```python
from build123d import *

# Parameters (mm, degrees)
REVOLVE1_ANGLE = 180


with BuildPart() as part:
    # Sketch1 → Revolve1 (revolve)
    with BuildSketch(Plane(origin=(0, 0, 0), x_dir=(1, 0, 0), z_dir=(0, 1, 0))):
        with BuildLine():
            Line((0, -6.35), (0, 6.35))
            Line((0, 6.35), (26.797, 6.35))
            ThreePointArc((26.797, 6.35), (27.695025612, 5.978025612), (28.067, 5.08))
            Line((28.067, 5.08), (28.067, 4.787411514))
            ThreePointArc((28.067, 4.787411514), (27.803594283, 4.013029212), (27.122641026, 3.5598701))
            ThreePointArc((27.122641026, 3.5598701), (24.384, 0), (27.122641026, -3.5598701))
            ThreePointArc((27.122641026, -3.5598701), (27.803594283, -4.013029212), (28.067, -4.787411514))
            Line((28.067, -4.787411514), (28.067, -5.08))
            ThreePointArc((28.067, -5.08), (27.695025612, -5.978025612), (26.797, -6.35))
            Line((26.797, -6.35), (0, -6.35))
        make_face()
    revolve(axis=Axis((0, 0, 6.35), (0, 0, -1)), revolution_arc=REVOLVE1_ANGLE)


solid = part.part
```
Can you work these out from the model? Positions are in its coordinate system, mm. Coordinates: 2 decimals unless noted, no trailing zeros. Write each loop counter-clockwise with the first axis right and the second up, starting at its lowest first coordinate (ties: lowest second). Pieces come first, ordered by that corner, then holes. Notation, with made-up numbers: M 64,69.5 L 114,69.5 A15 cw 114,81.5 Z; hole C 78,82.25 d4. An arc over 180 degrees is marked long. Write item = value, one per line. Start each with the question number.
Q1. If we section it at B-B, the plane z = -2.75: Write out the boundary of the cut face in (x, y), then the cut area to 3 significant figures.
Q2. If we section it at C-C, the plane z = 4.25: Write out the boundary of the cut face in (x, y).
Q3. If I drill on L1, parallel to Y at x = -19.5, z = 4.5; L2, parallel to Y at x = -1.5, z = -2.5; L3, parallel to X at y = -2, z = 2, over which ranges is the centre line in solid material (lowest first)? Write a range as [from, to].
Q4. I'm going to push flat-ended pins straight in: pin 1 (10 mm diameter, centred on x = 19, y = -23, fed in from +Z); pin 2 (4 mm diameter, centred on y = -6.5, z = -0.5, fed in from +X); pin 3 (3 mm diameter, centred on y = -10, z = 3.5, fed in from +X). Where does each tip first touch, or does it pass through?
Q5. If we section it at A-A, the plane x = 0: Write out the boundary of the cut face in (y, z).
Check sheet entries:
q1.outline = M -25.62,0 A25.62 ccw 25.62,0 Z
q1.area = 1,030 mm²
q2.outline = M -27.95,0 A27.95 ccw 27.95,0 Z
q3.L1 = [-20.14, 0]
q3.L2 = [-25.32, 0]
q3.L3 = [-24.89, 24.89]
q4.pin_1 = 6.35
q4.pin_2 = 24.58
q4.pin_3 = 26.59
q5.outline = M -28.07,-5.08 A1.27 ccw -26.8,-6.35 L 0,-6.35 L 0,6.35 L -26.8,6.35 A1.27 ccw -28.07,5.08 L -28.07,4.79 A1.27 ccw -27.12,3.56 A3.68 cw -27.12,-3.56 A1.27 ccw -28.07,-4.79 Z
